```python
from build123d import *

# Parameters (mm, degrees)
F0_W      = 25
F0_H      = 25
F0_R      = 1.5
F1_DEPTH  = 3
F3_DEPTH  = 5
F4_W      = 6
F4_H      = 12.5
F4_W_2    = 12.5
F4_H_2    = 6
F5_DEPTH  = 10
F7_DEPTH  = 4
F8_R      = 1.7
F9_DEPTH  = 25
F11_DEPTH = 4
F12_R     = 1.7
F13_DEPTH = 25


with BuildPart() as f1:
    # F0 (on Front) → F1 (new body)
    with BuildSketch(Plane.XZ):
        Rectangle(F0_W, F0_H)
        with Locations((-8.5, -7.5)):
            Circle(F0_R, mode=Mode.SUBTRACT)
    extrude(amount=F1_DEPTH)

    # F2 (on Front) → F3 (join)
    with BuildSketch(Plane.XZ):
        Polygon((-12.5, -12.5), (-12.5, 12.5), (-15.5, 12.5), (-15.5, -15.5), (12.5, -15.5), (12.5, -12.5), align=None)
    extrude(amount=F3_DEPTH)

    # F4 (on face) → F5 (join)
    with BuildSketch(Plane(origin=(0, 0, 0), x_dir=(-1, 0, 0), z_dir=(0, 1, 0))):
        with Locations((12.5, 6.25)):
            Rectangle(F4_W, F4_H)
        with Locations((-6.25, -12.5)):
            Rectangle(F4_W_2, F4_H_2)
    extrude(amount=F5_DEPTH)

    # F6 (on face) → F7 (cut)
    with BuildSketch(Plane.XY.offset(-9.5)):
        Polygon((8.097521, 1.8), (9.945042, 5), (8.097521, 8.2), (4.402479, 8.2), (2.554958, 5), (4.402479, 1.8), align=None)
    extrude(amount=-F7_DEPTH, mode=Mode.SUBTRACT)

    # F8 (on face) → F9 (cut)
    with BuildSketch(Plane.XY.offset(-9.5)):
        with Locations((6.25, 5)):
            Circle(F8_R)
    extrude(amount=-F9_DEPTH, mode=Mode.SUBTRACT)

    # F10 (on face) → F11 (cut)
    with BuildSketch(Plane.YZ.offset(-9.5)):
        Polygon((8.2, 4.402479), (8.2, 8.097521), (5, 9.945042), (1.8, 8.097521), (1.8, 4.402479), (5, 2.554958), align=None)
    extrude(amount=-F11_DEPTH, mode=Mode.SUBTRACT)

    # F12 (on face) → F13 (cut)
    with BuildSketch(Plane.YZ.offset(-9.5)):
        with Locations((5, 6.25)):
            Circle(F12_R)
    extrude(amount=-F13_DEPTH, mode=Mode.SUBTRACT)


solid = f1.part
```
Geometry check sheet. Reference: the model listing, model coordinates, mm. A direction names the side the tool comes from. Give positions to 0.01 mm unless a question says otherwise; leave off trailing zeros. Write each loop counter-clockwise with the first axis right and the second up, starting at its lowest first coordinate (ties: lowest second). Pieces come first, ordered by that corner, then holes. Notation, with made-up numbers: (-8.5, 17) - (35.5, 17) arc R22 cw to (35.5, 26) - close; hole circle Ø1 at (42, 39.25). An arc over 180 degrees is marked (long way). Use a Markdown table: item, result.
Q1. Section check C-C, the plane y = 1.25. Enter the section's corners in (x, z).
Computed:
| item | result |
|---|---|
| outline | (-15.5, 0) - (-9.5, 0) - (-9.5, 12.5) - (-15.5, 12.5) - close; (0, -15.5) - (12.5, -15.5) - (12.5, -9.5) - (0, -9.5) - close |
Q2. Go/stop test with flat-tipped pins: P1, Ø3.5, axis at x = -8.5, z = -7.5, coming from the -Y side; P2, Ø5, axis at y = 3.5, z = 6, coming from the -X side; P3, Ø4.5, axis at y = 5, z = 6.25, coming from the +X side; P4, Ø2, axis at y = -4.5, z = 2.5, coming from the +X side. Record where each tip stops, or that it passes through.
Computed:
| item | result |
|---|---|
| P1 | stops at y = -3 |
| P2 | stops at x = -15.5 |
| P3 | stops at x = -13.5 |
| P4 | stops at x = -12.5 |
Q3. Section check D-D, the plane z = -10.25. Enter the section's corners in (x, y).
Computed:
| item | result |
|---|---|
| outline | (-15.5, -5) - (-12.5, -5) - (-12.5, -3) - (12.5, -3) - (12.5, 10) - (0, 10) - (0, 0) - (-15.5, 0) - close; hole (2.55, 5) - (4.4, 1.8) - (8.1, 1.8) - (9.95, 5) - (8.1, 8.2) - (4.4, 8.2) - close |
Q4. Thickness scan on L1, parallel to Y at x = 5.75, z = -11.5; L2, parallel to Z at x = 8.75, y = 3.25; L3, parallel to X at y = 7.75, z = 2. Record the ranges inside material, lowest first. Write a range as [from, to].
Computed:
| item | result |
|---|---|
| L1 | y = [-3, 1.8], [8.2, 10] |
| L2 | z = [-15.5, -13.5] |
| L3 | x = [-15.5, -9.5] |
Q5. Section check B-B, the plane z = 6.25. Enter the section's corners in (x, y), then the cut area to 3 significant figures.
Computed:
| item | result |
|---|---|
| outline | (-15.5, -5) - (-12.5, -5) - (-12.5, -3) - (12.5, -3) - (12.5, 0) - (-9.5, 0) - (-9.5, 1.8) - (-13.5, 1.8) - (-13.5, 3.3) - (-15.5, 3.3) - close; (-15.5, 6.7) - (-13.5, 6.7) - (-13.5, 8.2) - (-9.5, 8.2) - (-9.5, 10) - (-15.5, 10) - close |
| area | 118 mm² |
Q6. Section check A-A, the plane x = 6.25. Enter the section's corners in (y, z).
Computed:
| item | result |
|---|---|
| outline | (-5, -15.5) - (3.3, -15.5) - (3.3, -13.5) - (1.8, -13.5) - (1.8, -9.5) - (0, -9.5) - (0, 12.5) - (-3, 12.5) - (-3, -12.5) - (-5, -12.5) - close; (6.7, -15.5) - (10, -15.5) - (10, -9.5) - (8.2, -9.5) - (8.2, -13.5) - (6.7, -13.5) - close |
Q7. Set-up check for faces 5 (the face through (-9.5, 1.6, 6.2)), 6 (the face through (0, 5, -13)), 7 (the face through (6, 8.2, -11)), 8 (the face through (-12, 5, 0)), 9 (the face through (-11.472, 6.578, 3.466)): record each of +Z, -Z, +X, -X, +Y, -Y from which the full face is reachable in a straight line by a thin tool's end or side.
Computed:
| item | result |
|---|---|
| face 5 | +Z, -Z, +X, +Y |
| face 6 | +Z, -Z, -X, +Y |
| face 7 | +Z |
| face 8 | -Z, +X, -X, +Y |
| face 9 | +X |
Q8. Draft check along Y on faces 1 (the face through (9.01, 3.38, -11.47)), 2 (the face through (0, -3, 0)), 3 (the face through (6, 1.8, -11)), 4 (the face through (-12.5, -4, 0)). Enter one of: pulls with the +Y half, pulls with the -Y half, needs draft (parallel to the pull), parting line crosses it, or undercut.
Computed:
| item | result |
|---|---|
| face 1 | undercut |
| face 2 | pulls with the -Y half |
| face 3 | undercut |
| face 4 | needs draft |
